Part model, mm, in its own coordinate system. Face numbers are marked on the shaded views. A direction names the side the tool comes from. Coordinates: 2 decimals unless noted, no trailing zeros. Order: outer loops, then holes, each group sorted by start corner. A loop starts at its lowest first (then second) coordinate and runs counter-clockwise, first axis right, second up. Notation, with made-up numbers: M -23.5,13.5 L -8.5,13.5 A31 cw -8.5,45.5 Z; hole C 7,-10.75 d5. An arc over 180 degrees is marked long. Answer in a Markdown table with one row per item. Add a question column.
from build123d import *

# Parameters (mm, degrees)
SKETCH1_W           = 80
SKETCH1_H           = 50
SKETCH1_W_2         = 74
SKETCH1_H_2         = 44
BOSS_EXTRUDE1_DEPTH = 50
SKETCH2_R           = 2
SKETCH2_R_2         = 6
CUT_EXTRUDE1_DEPTH  = 3
CUT_EXTRUDE2_REACH  = 5
SKETCH3_R           = 2.5


with BuildPart() as part:
    # Sketch1 → Boss-Extrude1 (new body)
    with BuildSketch(Plane(origin=(0, 0, 0), x_dir=(1, 0, 0), z_dir=(0, 0, -1))):
        with Locations((40, 25)):
            Rectangle(SKETCH1_W, SKETCH1_H)
        with Locations((40, 25)):
            Rectangle(SKETCH1_W_2, SKETCH1_H_2, mode=Mode.SUBTRACT)
    extrude(amount=BOSS_EXTRUDE1_DEPTH)

    # Sketch2 → Cut-Extrude1 (cut)
    with BuildSketch(Plane(origin=(80, 0, 0), x_dir=(0, 0, -1), z_dir=(1, 0, 0))):
        with Locations((9.5, -25)):
            Circle(SKETCH2_R)
        with Locations((17.25, -38.423393759)):
            Circle(SKETCH2_R)
        with Locations((32.75, -38.423393759)):
            Circle(SKETCH2_R)
        with Locations((40.5, -25)):
            Circle(SKETCH2_R)
        with Locations((32.75, -11.576606241)):
            Circle(SKETCH2_R)
        with Locations((17.25, -11.576606241)):
            Circle(SKETCH2_R)
        with Locations((25, -32)):
            Circle(SKETCH2_R_2)
    extrude(amount=-CUT_EXTRUDE1_DEPTH, mode=Mode.SUBTRACT)

    # Sketch3 → Cut-Extrude2 (cut, up to next)
    with BuildSketch(Plane(origin=(3, 0, 0), x_dir=(0, 0, -1), z_dir=(1, 0, 0)), mode=Mode.PRIVATE) as cut_extrude2_sk1:
        with Locations((15, -40)):
            Circle(SKETCH3_R)
    cut_extrude2_tool1 = extrude(cut_extrude2_sk1.sketch, amount=-CUT_EXTRUDE2_REACH, mode=Mode.PRIVATE) & part.part
    add(cut_extrude2_tool1.solids().sort_by_distance((3, -40, -15))[0], mode=Mode.SUBTRACT)
    # Sketch3 → Cut-Extrude2 (cut, up to next)
    with BuildSketch(Plane(origin=(3, 0, 0), x_dir=(0, 0, -1), z_dir=(1, 0, 0)), mode=Mode.PRIVATE) as cut_extrude2_sk2:
        with Locations((15, -10)):
            Circle(SKETCH3_R)
    cut_extrude2_tool2 = extrude(cut_extrude2_sk2.sketch, amount=-CUT_EXTRUDE2_REACH, mode=Mode.PRIVATE) & part.part
    add(cut_extrude2_tool2.solids().sort_by_distance((3, -10, -15))[0], mode=Mode.SUBTRACT)
    # Sketch3 → Cut-Extrude2 (cut, up to next)
    with BuildSketch(Plane(origin=(3, 0, 0), x_dir=(0, 0, -1), z_dir=(1, 0, 0)), mode=Mode.PRIVATE) as cut_extrude2_sk3:
        with Locations((35, -10)):
            Circle(SKETCH3_R)
    cut_extrude2_tool3 = extrude(cut_extrude2_sk3.sketch, amount=-CUT_EXTRUDE2_REACH, mode=Mode.PRIVATE) & part.part
    add(cut_extrude2_tool3.solids().sort_by_distance((3, -10, -35))[0], mode=Mode.SUBTRACT)
    # Sketch3 → Cut-Extrude2 (cut, up to next)
    with BuildSketch(Plane(origin=(3, 0, 0), x_dir=(0, 0, -1), z_dir=(1, 0, 0)), mode=Mode.PRIVATE) as cut_extrude2_sk4:
        with Locations((35, -40)):
            Circle(SKETCH3_R)
    cut_extrude2_tool4 = extrude(cut_extrude2_sk4.sketch, amount=-CUT_EXTRUDE2_REACH, mode=Mode.PRIVATE) & part.part
    add(cut_extrude2_tool4.solids().sort_by_distance((3, -40, -35))[0], mode=Mode.SUBTRACT)


solid = part.part
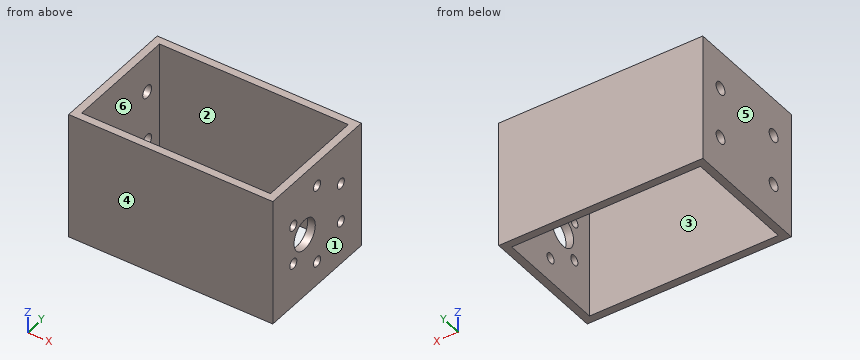
(1) Pull direction Y, two halves, no side cores. Call the marked faces 1, 2, 3 and 4: pulls with the +Y half, pulls with the -Y half, needs draft (parallel to the pull), parting line crosses it, or undercut.
(2) Slice it at B-B (y = -25). List the corners of the cut face in (x, z).
(3) Wall check: line 1 (Y direction, x = 79, z = -17); line 2 (Y direction, x = 0.9, z = -35); line 3 (Y direction, x = 16, z = -40). Give the ranges that are in metal, low to high.
(4) 3-axis set-ups, long thin cutter, end or side, ignore diameter. For the marked faces 5 and 6: which of +Z, -Z, +X, -X, +Y, -Y reach the whole face in a straight line?
(5) Slice it at A-A (x = 13.5). List the corners of the cut face in (y, z).
(6) Drop flat-ended pins along their axis: P1, Ø10, axis at x = 11.5, y = -12, coming from the -Z side; P2, Ø2, axis at x = 30.5, z = -24, coming from the +Y side; P3, Ø2.5, axis at y = -38.42, z = -17.25, coming from the +X side; P4, Ø3, axis at y = -40, z = -35, coming from the -X side. Give the stop position or say it passes through.
(7) Slice it at D-D (z = -25). List the corners of the cut face in (x, y).
(8) Slice it at C-C (z = -5). List the corners of the cut face in (x, y), and give its area (3 significant figures).
Computed:
| question | item | result |
|---|---|---|
| 1 | face 1 | needs draft |
| 1 | face 2 | undercut |
| 1 | face 3 | undercut |
| 1 | face 4 | pulls with the -Y half |
| 2 | outline | M 0,-50 L 3,-50 L 3,0 L 0,0 Z; M 77,-50 L 80,-50 L 80,-42.5 L 77,-42.5 Z; M 77,-38.5 L 80,-38.5 L 80,-11.5 L 77,-11.5 Z; M 77,-7.5 L 80,-7.5 L 80,0 L 77,0 Z |
| 3 | line 1 | y = -50 to -40.41, -36.44 to -13.56, -9.59 to 0 |
| 3 | line 2 | y = -50 to -42.5, -37.5 to -12.5, -7.5 to 0 |
| 3 | line 3 | y = -50 to -47, -3 to 0 |
| 4 | face 5 | +Z, -Z, -X, +Y, -Y |
| 4 | face 6 | +Z, -Z |
| 5 | outline | M -50,-50 L -47,-50 L -47,0 L -50,0 Z; M -3,-50 L 0,-50 L 0,0 L -3,0 Z |
| 6 | P1 | passes through |
| 6 | P2 | stops at y = 0 |
| 6 | P3 | stops at x = 3 |
| 6 | P4 | stops at x = 77 |
| 7 | outline | M 0,-50 L 80,-50 L 80,-38 L 77,-38 L 77,-47 L 3,-47 L 3,-3 L 77,-3 L 77,-26 L 80,-26 L 80,0 L 0,0 Z |
| 8 | outline | M 0,-50 L 80,-50 L 80,0 L 0,0 Z; hole M 3,-47 L 77,-47 L 77,-3 L 3,-3 Z |
| 8 | area | 744 mm^2 |
